Check sheet for the modelled part. Datum: model origin and axes. Units: mm. A direction names the side the tool comes from. Give positions to 0.01 mm unless a question says otherwise; leave off trailing zeros. Loops run counter-clockwise (first coordinate to the right, second up) from the corner with the lowest first, then second, coordinate; pieces in that order, holes last.
```python
from build123d import *

# Parameters (mm, degrees)
SKETCH_1_W          = 55
SKETCH_1_H          = 70
EXTRUDE_1_DEPTH     = 3
SKETCH_3_R          = 13
CUT_EXTRUDE_1_DEPTH = 45.612218057
SKETCH_4_R          = 1.5
CUT_EXTRUDE_2_DEPTH = 45.612218057
SKETCH_5_W          = 3
SKETCH_5_H          = 20
EXTRUDE_2_DEPTH     = 3
FILLET_1_R          = 1
FILLET_2_R          = 25
SKETCH_6_R          = 2
CUT_EXTRUDE_3_DEPTH = 47.521500406


with BuildPart() as part:
    # 草图1 → 凸台-拉伸1 (new body)
    with BuildSketch(Plane.XY):
        Rectangle(SKETCH_1_W, SKETCH_1_H)
    extrude(amount=EXTRUDE_1_DEPTH)

    # 草图3 → 切除-拉伸1 (cut, through all)
    with BuildSketch(Plane(origin=(0, 0, 0), x_dir=(-1, 0, 0), z_dir=(0, 0, -1))):
        with Locations((2.5, 0)):
            Circle(SKETCH_3_R)
    extrude(amount=-CUT_EXTRUDE_1_DEPTH, mode=Mode.SUBTRACT)

    # 草图4 → 切除-拉伸2 (cut, through all)
    with BuildSketch(Plane.XY.offset(3)):
        with Locations((24.5, 32)):
            Circle(SKETCH_4_R)
        with Locations((24.5, 22)):
            Circle(SKETCH_4_R)
        with Locations(Location((24.5, -22, 0), (0, 0, 180))):
            Circle(SKETCH_4_R)
        with Locations(Location((24.5, -32, 0), (0, 0, 180))):
            Circle(SKETCH_4_R)
    extrude(amount=-CUT_EXTRUDE_2_DEPTH, mode=Mode.SUBTRACT)

    # 草图5 → 凸台-拉伸2 (add)
    with BuildSketch(Plane.XY.offset(3)):
        with Locations((29, 0)):
            Rectangle(SKETCH_5_W, SKETCH_5_H)
    extrude(amount=-EXTRUDE_2_DEPTH)

    # 圆角1
    fillet_1_edges = [part.edges().sort_by_distance(p)[0] for p in [
        (30.5, 10, 1.5),
        (30.5, -10, 1.5),
        (27.5, -35, 1.5),
        (27.5, 35, 1.5),
    ]]
    fillet(fillet_1_edges, radius=FILLET_1_R)

    # 圆角2
    fillet_2_edges = [part.edges().sort_by_distance(p)[0] for p in [
        (-27.5, -35, 1.5),
        (-27.5, 35, 1.5),
    ]]
    fillet(fillet_2_edges, radius=FILLET_2_R)

    # 草图6 → 切除-拉伸3 (cut, through all)
    with BuildSketch(Plane(origin=(0, 0, 0), x_dir=(-1, 0, 0), z_dir=(0, 0, -1))):
        with Locations((17.5, 15)):
            Circle(SKETCH_6_R)
        with Locations(Location((17.5, -15, 0), (0, 0, 180))):
            Circle(SKETCH_6_R)
    extrude(amount=-CUT_EXTRUDE_3_DEPTH, mode=Mode.SUBTRACT)


solid = part.part
```
(1) Section check B-B on x = -17.5. Record the boundary of the cut face in (y, z).
(2) Section check C-C on y = -22. Record the boundary of the cut face in (x, z).
(3) Gauge pin test, flat ends, axial feed: pin 1 Ø1 at (x, z) = (28.5, 2) entering from +Y; pin 2 Ø1 at (x, z) = (28.5, 2) entering from -Y; pin 3 Ø0.9 at (y, z) = (25, 2) entering from +X. Record the tip position at first contact, or that the pin passes through.
(4) Access from +Z, -Z, +X, -X, +Y, -Y to the whole of each face (thin tool, end or side, straight path). Record for faces 1 (the face through (27.5, 22, 1)), 2 (the face through (23.39, 23.01, 1.52)), 3 (the face through (28, -10, 2)).
(5) Release check for a two-part mould opening along X. For faces 4 (the face through (12, -35, 1)), 5 (the face through (-17.24, 16.983, 1.479)), 6 (the face through (-20.371, 27.482, 1.521)), 7 (the face through (-17.76, -16.983, 1.479)) record: pulls with the +X half, pulls with the -X half, needs draft (parallel to the pull), parting line crosses it, or undercut.
(6) Material ranges on line 1 (Y direction, x = 24.5, z = 1.5); line 2 (Y direction, x = -2.5, z = 1.85); line 3 (Y direction, x = -17.5, z = 1.15), recorded low to high.
(7) Section check D-D on x = 2. Record the boundary of the cut face in (y, z), plus the area to 3 significant figures.
(8) Section check A-A on x = 24.5. Record the boundary of the cut face in (y, z).
Computed values:
1. outline: (-30, 0) - (-17, 0) - (-17, 3) - (-30, 3) - close; (-13, 0) - (13, 0) - (13, 3) - (-13, 3) - close; (17, 0) - (30, 0) - (30, 3) - (17, 3) - close
2. outline: (-24.43, 0) - (23, 0) - (23, 3) - (-24.43, 3) - close; (26, 0) - (27.5, 0) - (27.5, 3) - (26, 3) - close
3. pin 1: stops at y = 10
3. pin 2: stops at y = -10
3. pin 3: stops at x = 27.5
4. face 1: +Z, -Z, +X, +Y
4. face 2: +Z, -Z
4. face 3: +Z, -Z, +X, -Y
5. face 4: needs draft
5. face 5: undercut
5. face 6: pulls with the -X half
5. face 7: undercut
6. line 1: y = -35 to -33.5, -30.5 to -23.5, -20.5 to 20.5, 23.5 to 30.5, 33.5 to 35
6. line 2: y = -35 to -13, 13 to 35
6. line 3: y = -30 to -17, -13 to 13, 17 to 30
7. outline: (-35, 0) - (-12.2, 0) - (-12.2, 3) - (-35, 3) - close; (12.2, 0) - (35, 0) - (35, 3) - (12.2, 3) - close
7. area: 137 mm2
8. outline: (-35, 0) - (-33.5, 0) - (-33.5, 3) - (-35, 3) - close; (-30.5, 0) - (-23.5, 0) - (-23.5, 3) - (-30.5, 3) - close; (-20.5, 0) - (20.5, 0) - (20.5, 3) - (-20.5, 3) - close; (23.5, 0) - (30.5, 0) - (30.5, 3) - (23.5, 3) - close; (33.5, 0) - (35, 0) - (35, 3) - (33.5, 3) - close
